Can you work these out from the model? Positions are in its coordinate system, mm. A direction names the side the tool comes from. Give positions to 0.01 mm unless a question says otherwise; leave off trailing zeros. Write each loop counter-clockwise with the first axis right and the second up, starting at its lowest first coordinate (ties: lowest second). Pieces come first, ordered by that corner, then holes. Notation, with made-up numbers: M 86,86.25 L 90,86.25 A7 ccw 90,96.25 Z; hole C -11.5,-30 d3. An arc over 180 degrees is marked long. Use CSV: the item, a comma, the result in double quotes. Start each with the question number.
from build123d import *

# Parameters (mm, degrees)
EXTRUDE_1_DEPTH = 4


with BuildPart() as part:
    # Sketch 1 → Бобышка-Вытянуть1 (new body)
    with BuildSketch(Plane(origin=(0, 18.459650088, -6.591530499), x_dir=(-8.942452936584094e-15, -0.6354457681716477, 0.7721455016463832), z_dir=(1, 0, 0))):
        Polygon((0, 0), (20.017301467, -2.12709708), (39.702713782, 0), (21.972488377, 21.671158416), (17.729847698, 21.671467431), align=None)
        Polygon((20.003340082, -0.12714581), (29.833488484, 9.841213252), (19.865129422, 19.671361654), (10.03498102, 9.703002592), align=None, mode=Mode.SUBTRACT)
    extrude(amount=EXTRUDE_1_DEPTH)


solid = part.part
(1) Please list where these lines run through material, in increasing order: L1, parallel to Z at x = 0.8, y = -1.5; L2, parallel to Y at x = 3.85, z = 6.5; L3, parallel to Z at x = 3.15, y = -6. Write a range as [from, to].
(2) I want a section at B-B (y = 2). Write out the boundary of the cut face in (x, z).
(3) I want a section at D-D (z = 17.5). Write out the boundary of the cut face in (x, y).
(4) Will these pins go through, and if not, where does the flat tip stop? pin 1 Ø2 at (x, z) = (1.5, 12) entering from +Y; pin 2 Ø1 at (x, y) = (3, -2.5) entering from -Z.
(5) Which directions (+Z, -Z, +X, -X, +Y, -Y) give clear straight access to the entire face, cutting with the end or side of a thin tool? Please do faces 1 (the face through (1.97, 13, 1.69)), 2 (the face through (1.97, 5.21, 1.87)).
(6) I want a section at C-C (z = -3). Write out the boundary of the cut face in (x, y).
(7) Thinking about a two-plate mould opening in Z: for faces 3 (the face through (1.972, -9.464, 10.526)), 4 (the face through (1.972, -8.716, 3.317)), 5 (the face through (1.97, -10.91, -5.01)), which applies, released by +Z, released by -Z, zero draft, split by the parting line, or undercut?
(8) I want a section at A-A (x = 3.6). Write out the boundary of the cut face in (y, z).
Geometry results:
1,L1,"z = [-6.65, -4.46], [9.6, 18.91]"
1,L2,"y = [-10.27, -8.43], [5.63, 9.83]"
1,L3,"z = [-6.66, -4.05], [10, 23.31]"
2,outline,"M 0,-6.64 L 4,-6.64 L 4,-4.78 L 0,-4.78 Z; M 0,9.28 L 4,9.28 L 4,15.48 L 0,15.48 Z"
3,outline,"M 0,-8.08 L 4,-8.08 L 4,-0.06 L 0,-0.06 Z"
4,pin 1,"stops at y = 6.58"
4,pin 2,"stops at z = -6.65"
5,face 1,"+Z, +X, -X, +Y"
5,face 2,"+X, -X"
6,outline,"M 0,-12.16 L 4,-12.16 L 4,-9.28 L 0,-9.28 Z; M 0,4.77 L 4,4.77 L 4,16.09 L 0,16.09 Z"
7,face 3,"released by +Z"
7,face 4,"undercut"
7,face 5,"released by -Z"
8,outline,"M -12.24,-3.4 L -9.54,-6.67 L 18.46,-6.59 L 7.38,10.22 L -6.77,24.06 Z; hole M -9.35,-3.75 L 4.59,-5.01 L 5.85,8.93 L -8.1,10.19 Z"
